Build history of the part. All positions in model axes, mm. Give positions to 0.01 mm unless a question says otherwise; leave off trailing zeros. Order: outer loops, then holes, each group sorted by start corner. A loop starts at its lowest first (then second) coordinate and runs counter-clockwise, first axis right, second up. Notation, with made-up numbers: M 81,13.25 L 111,13.25 A15 ccw 111,26.25 Z; hole C -19,86 d7. An arc over 180 degrees is marked long. One line per item, written item: value.
from build123d import *

# Parameters (mm, degrees)
SKETCH_1_W          = 14.3
SKETCH_1_H          = 25
SKETCH_1_W_2        = 25
SKETCH_1_H_2        = 14.3
EXTRUDE_1_DEPTH     = 7
FILLET_1_R          = 3
FILLET_3_R          = 23
EXTRUDE_START       = -7
EXTRUDE_2_DEPTH     = 7
SKETCH_7_R          = 1.75
CUT_EXTRUDE_5_DEPTH = 95.023294986
SKETCH_9_W          = 3
SKETCH_9_H          = 50
EXTRUDE_3_DEPTH     = 7
SKETCH_10_W         = 50
SKETCH_10_H         = 3
EXTRUDE_4_DEPTH     = 5
SKETCH_11_R         = 2.1
CUT_EXTRUDE_6_DEPTH = 104.928485027
SKETCH_12_R         = 2.1
CUT_EXTRUDE_7_DEPTH = 104.928485103


with BuildPart() as part:
    # 스케치1 → 보스-돌출1 (new body)
    with BuildSketch(Plane(origin=(0, 0, 0), x_dir=(1, 0, 0), z_dir=(0, 1, 0))):
        Polygon((-26, 52), (-39, 39), (-26, 39), (26, 39), (39, 39), (26, 52), (12.5, 52), (-12.5, 52), align=None)
        Polygon((-26, 39), (-39, 39), (-39, 26), align=None)
        Polygon((-39, 26), (-39, 39), (-52, 26), (-52, 12.5), (-52, -12.5), (-52, -26), (-39, -39), (-39, -26), align=None)
        with Locations((-59.15, 0)):
            Rectangle(SKETCH_1_W, SKETCH_1_H)
        with Locations((0, 59.15)):
            Rectangle(SKETCH_1_W_2, SKETCH_1_H_2)
        Polygon((39, 39), (26, 39), (39, 26), align=None)
        Polygon((52, 26), (39, 39), (39, 26), (39, -26), (39, -39), (52, -26), (52, -12.5), (52, 12.5), align=None)
        with Locations((59.15, 0)):
            Rectangle(SKETCH_1_W, SKETCH_1_H)
        Polygon((39, -39), (39, -26), (26, -39), align=None)
        Polygon((-26, -39), (-39, -39), (-26, -52), (-12.5, -52), (12.5, -52), (26, -52), (39, -39), (26, -39), align=None)
        Polygon((-26, -39), (-39, -26), (-39, -39), align=None)
        with Locations((0, -59.15)):
            Rectangle(SKETCH_1_W_2, SKETCH_1_H_2)
    extrude(amount=EXTRUDE_1_DEPTH)

    # 필렛1
    fillet_1_edges = [part.edges().sort_by_distance(p)[0] for p in [
        (12.5, 3.5, 66.3),
        (-12.5, 3.5, 66.3),
        (-66.3, 3.5, 12.5),
        (-66.3, 3.5, -12.5),
        (-12.5, 3.5, -66.3),
        (12.5, 3.5, -66.3),
        (66.3, 3.5, -12.5),
        (66.3, 3.5, 12.5),
    ]]
    fillet(fillet_1_edges, radius=FILLET_1_R)

    # 필렛3
    # the kernel refuses this fillet: 23 mm, written as the material it adds along each edge
    with BuildSketch(Plane(origin=(-39, 0, 26), x_dir=(0, 0, -1), z_dir=(0, 1, 0))) as fillet_3_piece_1:
        with BuildLine():
            CenterArc((FILLET_3_R * 0.414213562373, -FILLET_3_R), FILLET_3_R, 90, 45)
            Line((-FILLET_3_R * 0.292893218813, -FILLET_3_R * 0.292893218813), (0, 0))
            Line((0, 0), (FILLET_3_R * 0.414213562373, 0))
        make_face()
    extrude(amount=7)
    with BuildSketch(Plane(origin=(-26, 0, 39), x_dir=(1, 0, 0), z_dir=(0, 1, 0)), Plane(origin=(26, 0, 39), x_dir=(0.7071067811865479, 0, -0.7071067811865471), z_dir=(0, 1, 0)), Plane(origin=(39, 0, 26), x_dir=(0, 0, -1), z_dir=(0, 1, 0)), Plane(origin=(39, 0, -26), x_dir=(-0.7071067811865476, 0, -0.7071067811865476), z_dir=(0, 1, 0)), Plane(origin=(26, 0, -39), x_dir=(-1, 0, 0), z_dir=(0, 1, 0)), Plane(origin=(-26, 0, -39), x_dir=(-0.7071067811865471, 0, 0.7071067811865479), z_dir=(0, 1, 0)), Plane(origin=(-39, 0, -26), x_dir=(0, 0, 1), z_dir=(0, 1, 0))) as fillet_3_piece_2:
        with BuildLine():
            CenterArc((FILLET_3_R * 0.414213562373, FILLET_3_R), FILLET_3_R, 225, 45)
            Line((-FILLET_3_R * 0.292893218813, FILLET_3_R * 0.292893218813), (0, 0))
            Line((0, 0), (FILLET_3_R * 0.414213562373, 0))
        make_face()
    extrude(amount=7)

    # 스케치6 → 보스-돌출2 (add)
    with BuildSketch(Plane(origin=(0, 7, 0), x_dir=(1, 0, 0), z_dir=(0, 1, 0)).offset(EXTRUDE_START)):
        with BuildLine():
            Line((16.473088065, 39), (-16.473088065, 39))
            ThreePointArc((-16.473088065, 39), (-25.120040329, 37.312677367), (-32.4982797, 32.4982797))
            ThreePointArc((-32.4982797, 32.4982797), (-37.312677367, 25.120040329), (-39, 16.473088065))
            Line((-39, 16.473088065), (-39, -16.473088065))
            ThreePointArc((-39, -16.473088065), (-37.312677367, -25.120040329), (-32.4982797, -32.4982797))
            ThreePointArc((-32.4982797, -32.4982797), (-25.120040329, -37.312677367), (-16.473088065, -39))
            Line((-16.473088065, -39), (16.473088065, -39))
            ThreePointArc((16.473088065, -39), (25.120040329, -37.312677367), (32.4982797, -32.4982797))
            ThreePointArc((32.4982797, -32.4982797), (37.312677367, -25.120040329), (39, -16.473088065))
            Line((39, -16.473088065), (39, 16.473088065))
            ThreePointArc((39, 16.473088065), (37.312677367, 25.120040329), (32.4982797, 32.4982797))
            ThreePointArc((32.4982797, 32.4982797), (25.120040329, 37.312677367), (16.473088065, 39))
        make_face()
    extrude(amount=EXTRUDE_2_DEPTH)

    # 스케치7 → 컷-돌출5 (cut, through all)
    with BuildSketch(Plane(origin=(0, 7, 0), x_dir=(1, 0, 0), z_dir=(0, 1, 0))):
        with Locations(Location((0, 0, 0), (0, 0, 270))):
            Circle(SKETCH_7_R)
    extrude(amount=-CUT_EXTRUDE_5_DEPTH, mode=Mode.SUBTRACT)

    # 스케치9 → 보스-돌출3 (add)
    with BuildSketch(Plane(origin=(0, 7, 0), x_dir=(1, 0, 0), z_dir=(0, 1, 0))):
        with Locations((-44, 0)):
            Rectangle(SKETCH_9_W, SKETCH_9_H)
    extrude(amount=EXTRUDE_3_DEPTH)

    # 스케치10 → 보스-돌출4 (add)
    with BuildSketch(Plane(origin=(-42.5, 0, 0), x_dir=(0, 0, -1), z_dir=(1, 0, 0))):
        with Locations((0, 12.5)):
            Rectangle(SKETCH_10_W, SKETCH_10_H)
    extrude(amount=EXTRUDE_4_DEPTH)

    # 스케치11 → 컷-돌출6 (cut, through all)
    with BuildSketch(Plane.XY.offset(12.5)):
        with Locations(Location((-61.3, 3.5, 0), (0, 0, 197.752790162))):
            Circle(SKETCH_11_R)
        with Locations(Location((61.3, 3.5, 0), (0, 0, 17.752790162))):
            Circle(SKETCH_11_R)
    extrude(amount=-CUT_EXTRUDE_6_DEPTH, mode=Mode.SUBTRACT)

    # 스케치12 → 컷-돌출7 (cut, through all)
    with BuildSketch(Plane.ZY.offset(12.5)):
        with Locations(Location((-61.3, 3.5, 0), (0, 0, 162.247209838))):
            Circle(SKETCH_12_R)
        with Locations(Location((61.3, 3.5, 0), (0, 0, 17.752790162))):
            Circle(SKETCH_12_R)
    extrude(amount=-CUT_EXTRUDE_7_DEPTH, mode=Mode.SUBTRACT)


solid = part.part
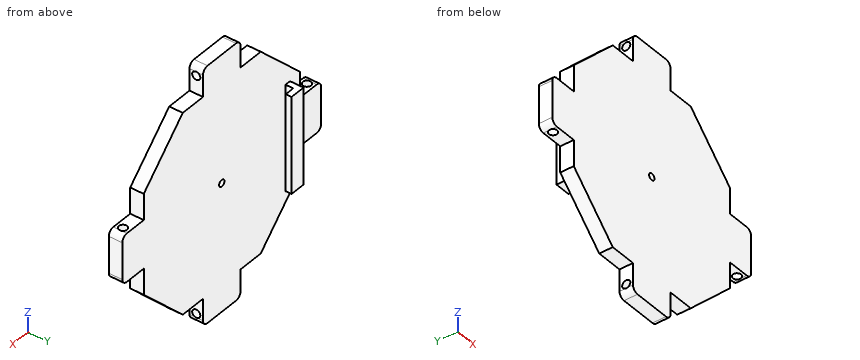
1) Saw through at A-A, the plane z = -61.3. Write the cut outline in (x, y), then the cut area to 3 significant figures.
Check values:
outline: M -12.5,0 L 12.5,0 L 12.5,1.4 L -12.5,1.4 Z; M -12.5,5.6 L 12.5,5.6 L 12.5,7 L -12.5,7 Z
area: 70.0 mm^2
2) Pin check, flat tips, straight feed: pin 1 (5 mm diameter, centred on x = -61.3, y = 3.5, fed in from -Z); pin 2 (2 mm diameter, centred on x = -40.5, y = 10.5, fed in from -Z); pin 3 (2 mm diameter, centred on x = -17.5, y = 2, fed in from +Z); pin 4 (3 mm diameter, centred on x = 0, z = 0, fed in from -Y). Stop position of each tip, or through.
Check values:
pin 1: z = -12.5
pin 2: z = -25
pin 3: z = 52
pin 4: through
3) Saw through at D-D, the plane z = 16. Write the cut outline in (x, y).
Check values:
outline: M -52,0 L 52,0 L 52,7 L -42.5,7 L -42.5,11 L -37.5,11 L -37.5,14 L -45.5,14 L -45.5,7 L -52,7 Z
4) Drill centre lines: probe 1 along X at (y, z) = (2.5, -6.5); probe 2 along Y at (x, z) = (61, 0); probe 3 along X at (y, z) = (7.25, -3.5). Where is each one in solid material? Low to high. Write a range as from..to.
Check values:
probe 1: -66.3..-63.15, -59.45..59.45, 63.15..66.3
probe 2: 0..1.42, 5.58..7
probe 3: -45.5..-42.5
5) Saw through at C-C, the plane z = 0. Write the cut outline in (x, y), then the cut area to 3 significant figures.
Check values:
outline: M -66.3,0 L -1.75,0 L -1.75,7 L -42.5,7 L -42.5,11 L -37.5,11 L -37.5,14 L -45.5,14 L -45.5,7 L -66.3,7 Z; M 1.75,0 L 66.3,0 L 66.3,7 L 1.75,7 Z; hole C -61.3,3.5 d4.2; hole C 61.3,3.5 d4.2
area: 912 mm^2
6) Saw through at B-B, the plane x = 61.3. Write the cut outline in (y, z), then the cut area to 3 significant figures.
Check values:
outline: M 0,-12.5 L 1.4,-12.5 L 1.4,12.5 L 0,12.5 Z; M 5.6,-12.5 L 7,-12.5 L 7,12.5 L 5.6,12.5 Z
area: 70.0 mm^2
